from build123d import *

# Parameters (mm, degrees)
F0_W     = 57
F0_H     = 60
F0_R     = 2.55
F1_DEPTH = 2.5
F2_W     = 57
F2_H     = 2
F3_DEPTH = 7
F5_R     = 2.55
F6_DEPTH = 2


with BuildPart() as f1:
    # F0 (on Front) → F1 (new body, symmetric)
    with BuildSketch(Plane.XZ):
        with Locations((-26.5, 28.9)):
            Rectangle(F0_W, F0_H)
        with Locations((-42.45, 9.45)):
            Circle(F0_R, mode=Mode.SUBTRACT)
        with Locations((-8.55, 9.45)):
            Circle(F0_R, mode=Mode.SUBTRACT)
        with Locations((-42.45, 48.35)):
            Circle(F0_R, mode=Mode.SUBTRACT)
        with Locations((-8.55, 48.35)):
            Circle(F0_R, mode=Mode.SUBTRACT)
    extrude(amount=F1_DEPTH, both=True)

    # F2 (on face) → F3 (join)
    with BuildSketch(Plane.XZ.offset(2.5)):
        with Locations((-26.5, 59.9)):
            Rectangle(F2_W, F2_H)
        with Locations((-26.5, -2.1)):
            Rectangle(F2_W, F2_H)
    extrude(amount=-F3_DEPTH)

    # F5 (on face) → F6 (cut)
    with BuildSketch(Plane(origin=(0, 2.5, 0), x_dir=(-1, 0, 0), z_dir=(0, 1, 0))):
        Polygon((40.490779, 6.056529), (44.409221, 6.056529), (46.368442, 9.45), (44.409221, 12.843471), (40.490779, 12.843471), (38.531558, 9.45), align=None)
        with Locations((42.45, 9.45)):
            Circle(F5_R, mode=Mode.SUBTRACT)
        Polygon((6.590779, 6.056529), (10.509221, 6.056529), (12.468442, 9.45), (10.509221, 12.843471), (6.590779, 12.843471), (4.631558, 9.45), align=None)
        with Locations((8.55, 9.45)):
            Circle(F5_R, mode=Mode.SUBTRACT)
        Polygon((6.444065, 44.702414), (10.655935, 44.702414), (12.761869, 48.35), (10.655935, 51.997586), (6.444065, 51.997586), (4.338131, 48.35), align=None)
        with Locations((8.55, 48.35)):
            Circle(F5_R, mode=Mode.SUBTRACT)
        Polygon((40.344065, 44.702414), (44.555935, 44.702414), (46.661869, 48.35), (44.555935, 51.997586), (40.344065, 51.997586), (38.238131, 48.35), align=None)
        with Locations((42.45, 48.35)):
            Circle(F5_R, mode=Mode.SUBTRACT)
    extrude(amount=-F6_DEPTH, mode=Mode.SUBTRACT)


solid = f1.part
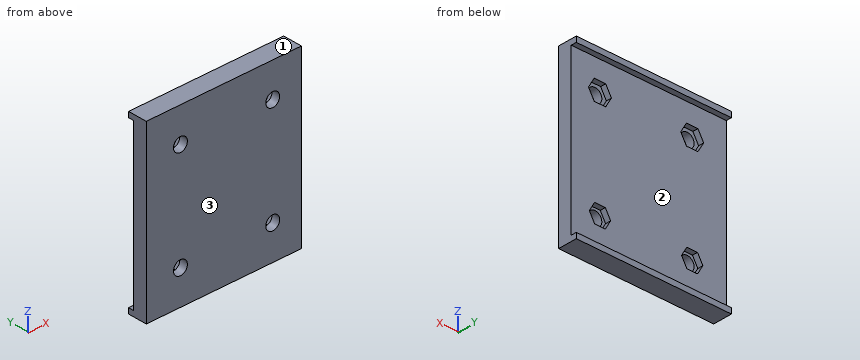
Could you check a few things on this model? Use its own coordinates, in mm. Face numbers are marked on the shaded views. Give positions to 0.01 mm unless a question says otherwise; leave off trailing zeros. Order: outer loops, then holes, each group sorted by start corner. A loop starts at its lowest first (then second) coordinate and runs counter-clockwise, first axis right, second up.
1. Suppose I cut it at D-D (z = 22). Write out the boundary of the cut face in (x, y).
Answers below:
outline: (-55, -2.5) - (2, -2.5) - (2, 2.5) - (-55, 2.5) - close
2. For pin 1 (8 mm diameter, centred on x = -10, z = 48, fed in from +Y); pin 2 (4.5 mm diameter, centred on x = -42.45, z = 9.45, fed in from -Y); pin 3 (3.5 mm diameter, centred on x = -44, z = 49, fed in from +Y), each with a flat end and sliding along its axis, tell me the tip position at first contact or that it passes through.
Answers below:
pin 1: stops at y = 2.5
pin 2: passes through
pin 3: stops at y = 0.5
3. Suppose I cut it at A-A (x = -42.45). Write out the boundary of the cut face in (y, z).
Answers below:
outline: (-2.5, -3.1) - (4.5, -3.1) - (4.5, -1.1) - (2.5, -1.1) - (2.5, 6.06) - (0.5, 6.06) - (0.5, 6.9) - (-2.5, 6.9) - close; (-2.5, 12) - (0.5, 12) - (0.5, 12.84) - (2.5, 12.84) - (2.5, 44.7) - (0.5, 44.7) - (0.5, 45.8) - (-2.5, 45.8) - close; (-2.5, 50.9) - (0.5, 50.9) - (0.5, 52) - (2.5, 52) - (2.5, 58.9) - (4.5, 58.9) - (4.5, 60.9) - (-2.5, 60.9) - close
4. Thinking about a two-plate mould opening in Z: for the marked faces 1, 2 and 3, which applies, +Z half, -Z half, draft (parallel to the pull), parting line (faces both ways), or undercut?
Answers below:
face 1: +Z half
face 2: undercut
face 3: draft
5. Suppose I cut it at B-B (y = -0.25). Write out the boundary of the cut face in (x, z).
Answers below:
outline: (-55, -3.1) - (2, -3.1) - (2, 60.9) - (-55, 60.9) - close; hole circle Ø5.1 at (-42.45, 9.45); hole circle Ø5.1 at (-42.45, 48.35); hole circle Ø5.1 at (-8.55, 9.45); hole circle Ø5.1 at (-8.55, 48.35)
6. I need wall thicknesses on L1, parallel to Z at x = -8.55, y = -1.5; L2, parallel to X at y = -0.4, z = 9.45; L3, parallel to Z at x = -8, y = 1. Which ranges of each line are inside material? Lowest first, please.
Answers below:
L1: z = -3.1 to 6.9, 12 to 45.8, 50.9 to 60.9
L2: x = -55 to -45, -39.9 to -11.1, -6 to 2
L3: z = -3.1 to 6.06, 12.84 to 44.7, 52 to 60.9
